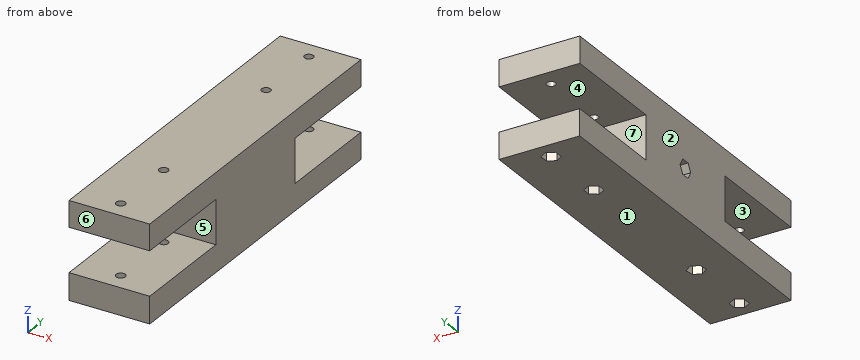
```python
from build123d import *

# Parameters (mm, degrees)
PAD_DEPTH            = 30
SKETCH001_R          = 1.647318
SKETCH001_R_2        = 1.644279
SKETCH001_R_3        = 1.702169
SKETCH001_R_4        = 1.703214
POCKET_DEPTH         = 600
POCKET_DEPTH_BACK    = -600
POCKET001_DEPTH      = 3.3
POCKET001_DEPTH_BACK = -3.3
SKETCH005_R          = 1.5
POCKET006_DEPTH      = 5
POCKET006_FACE59_R   = 1.5
POCKET007_DEPTH      = 5


with BuildPart() as part:
    # Sketch → Pad (new body)
    with BuildSketch(Plane.YZ.offset(707.5)):
        Polygon((-29.833706, -213.381088), (98.242805, -213.381088), (98.242805, -223.224411), (58.176593, -223.224411), (58.176593, -239.563995), (98.283882, -239.563995), (98.283882, -249.413437), (-29.832484, -249.413437), (-29.832484, -239.402665), (10.249295, -239.402665), (10.249295, -223.039155), (-29.833706, -223.039155), align=None)
    extrude(amount=-PAD_DEPTH)

    # Sketch001 (on Face1 of Pad) → Pocket (cut, two sides)
    with BuildSketch(Plane(origin=(707.5, 0, -213.381088), x_dir=(0, -1, 0), z_dir=(0, 0, 1))) as pocket_sk:
        with Locations((-91.299301, -15.072129)):
            Circle(SKETCH001_R)
        with Locations((-65.313827, -15.0565)):
            Circle(SKETCH001_R_2)
        with Locations((-3.04988, -14.977353)):
            Circle(SKETCH001_R_3)
        with Locations((22.941161, -14.98072)):
            Circle(SKETCH001_R_4)
    extrude(amount=-POCKET_DEPTH, mode=Mode.SUBTRACT)
    extrude(pocket_sk.sketch, amount=-POCKET_DEPTH_BACK, mode=Mode.SUBTRACT)

    # Sketch002 → Pocket001 (cut, two sides)
    with BuildSketch(Plane.XY.offset(-249.6)) as pocket001_sk:
        Polygon((689.718567, -21.348757), (689.712699, -24.584869), (692.51232, -26.208007), (695.317809, -24.595033), (695.323677, -21.358921), (692.524056, -19.735783), align=None)
        Polygon((689.964521, 5.02151), (689.5629, 1.806498), (692.146371, -0.148822), (695.131463, 1.11087), (695.533085, 4.325882), (692.949613, 6.281202), align=None)
        Polygon((689.710385, 63.575304), (692.575997, 62.063394), (695.318155, 63.789132), (695.194701, 67.026779), (692.32909, 68.538689), (689.586932, 66.812951), align=None)
        Polygon((689.714374, 93.046585), (689.545318, 89.810999), (692.262889, 88.046798), (695.149518, 89.518184), (695.318574, 92.75377), (692.601003, 94.517971), align=None)
    extrude(amount=-POCKET001_DEPTH, mode=Mode.SUBTRACT)
    extrude(pocket001_sk.sketch, amount=-POCKET001_DEPTH_BACK, mode=Mode.SUBTRACT)

    # Sketch005 (on Face4 of Pocket001) → Pocket006 (cut)
    with BuildSketch(Plane(origin=(677.5, 0, 0), x_dir=(0, 1, 0), z_dir=(-1, 0, 0))):
        Polygon((37.439188, 231.557562), (35.826938, 234.350061), (32.602438, 234.350061), (30.990188, 231.557562), (32.602438, 228.765063), (35.826938, 228.765063), align=None)
        with Locations((34.214688, 231.557562)):
            Circle(SKETCH005_R, mode=Mode.SUBTRACT)
    extrude(amount=-POCKET006_DEPTH, mode=Mode.SUBTRACT)

    # Pocket006 Face59 → Pocket007 (cut)
    with BuildSketch(Plane(origin=(677.5, 34.214688, -231.557562), x_dir=(0, 1, 0), z_dir=(-1, 0, 0))):
        Circle(POCKET006_FACE59_R)
    extrude(amount=-POCKET007_DEPTH, mode=Mode.SUBTRACT)


solid = part.part
```
Check sheet for the modelled part. Datum: model origin and axes. Units: mm. Face numbers are marked on the shaded views. A direction names the side the tool comes from. Coordinates: 2 decimals unless noted, no trailing zeros. Write each loop counter-clockwise with the first axis right and the second up, starting at its lowest first coordinate (ties: lowest second). Pieces come first, ordered by that corner, then holes. Notation, with made-up numbers: M 38.5,88 L 95.5,88 A12 ccw 95.5,104 Z; hole C 3.5,77.25 d5. An arc over 180 degrees is marked long. Write item = value, one per line. Start each with the question number.
1. Go/stop test with flat-tipped pins: pin 1 (2 mm diameter, centred on x = 692.43, y = 91.3, fed in from +Z); pin 2 (2 mm diameter, centred on x = 687.5, z = -237, fed in from +Y); pin 3 (5 mm diameter, centred on x = 696.5, z = -216, fed in from +Y); pin 4 (4.5 mm diameter, centred on y = 34.5, z = -231.5, fed in from -X). Record where each tip stops, or that it passes through.
2. Tool access check on the marked faces 5, 6 and 7. Record the directions out of +Z, -Z, +X, -X, +Y, -Y that give a thin tool (end or side, any length) a straight path to the whole face; none if there is none.
3. Sectioned sample at D-D (z = -227). Record the cut outline in (x, y), then the cut area to 3 significant figures.
4. Thickness scan on probe 1 along Z at (x, y) = (688, 67.5); probe 2 along Z at (x, y) = (696, 1); probe 3 along Y at (x, z) = (693.75, -218). Record the ranges inside material, lowest first.
5. Sectioned sample at A-A (y = -16.5). Record the cut outline in (x, z).
6. Sectioned sample at C-C (y = 60). Record the cut outline in (x, z), then the cut area to 3 significant figures.
7. Sectioned sample at B-B (x = 684). Record the cut outline in (y, z), then the cut area to 3 significant figures.
8. Mould release check, pull along Z, two halves, no side actions. Record for the marked faces 1, 2, 3 and 4: pulls with the +Z half, pulls with the -Z half, needs draft (parallel to the pull), parting line crosses it, or undercut.
The answers:
q1.pin_1 = through
q1.pin_2 = 58.18
q1.pin_3 = 98.24
q1.pin_4 = 682.5
q2.face_5 = +X, -X, -Y
q2.face_6 = +Z, -Z, +X, -X, -Y
q2.face_7 = +X, -X, +Y
q3.outline = M 677.5,10.25 L 707.5,10.25 L 707.5,58.18 L 677.5,58.18 Z
q3.area = 1,440 mm²
q4.probe_1 = -249.41 to -239.56, -223.22 to -213.38
q4.probe_2 = -249.41 to -239.4, -223.04 to -213.38
q4.probe_3 = -29.83 to -24.12, -21.76 to 1.87, 4.23 to 64.32, 66.31 to 90.32, 92.28 to 98.24
q5.outline = M 677.5,-249.41 L 707.5,-249.41 L 707.5,-239.4 L 677.5,-239.4 Z; M 677.5,-223.04 L 707.5,-223.04 L 707.5,-213.38 L 677.5,-213.38 Z
q6.outline = M 677.5,-249.41 L 707.5,-249.41 L 707.5,-239.56 L 677.5,-239.56 Z; M 677.5,-223.22 L 707.5,-223.22 L 707.5,-213.38 L 677.5,-213.38 Z
q6.area = 591 mm²
q7.outline = M -29.83,-249.41 L 98.28,-249.41 L 98.28,-239.56 L 58.18,-239.56 L 58.18,-223.22 L 98.24,-223.22 L 98.24,-213.38 L -29.83,-213.38 L -29.83,-223.04 L 10.25,-223.04 L 10.25,-239.4 L -29.83,-239.4 Z
q7.area = 3,300 mm²
q8.face_1 = pulls with the -Z half
q8.face_2 = needs draft
q8.face_3 = undercut
q8.face_4 = undercut
